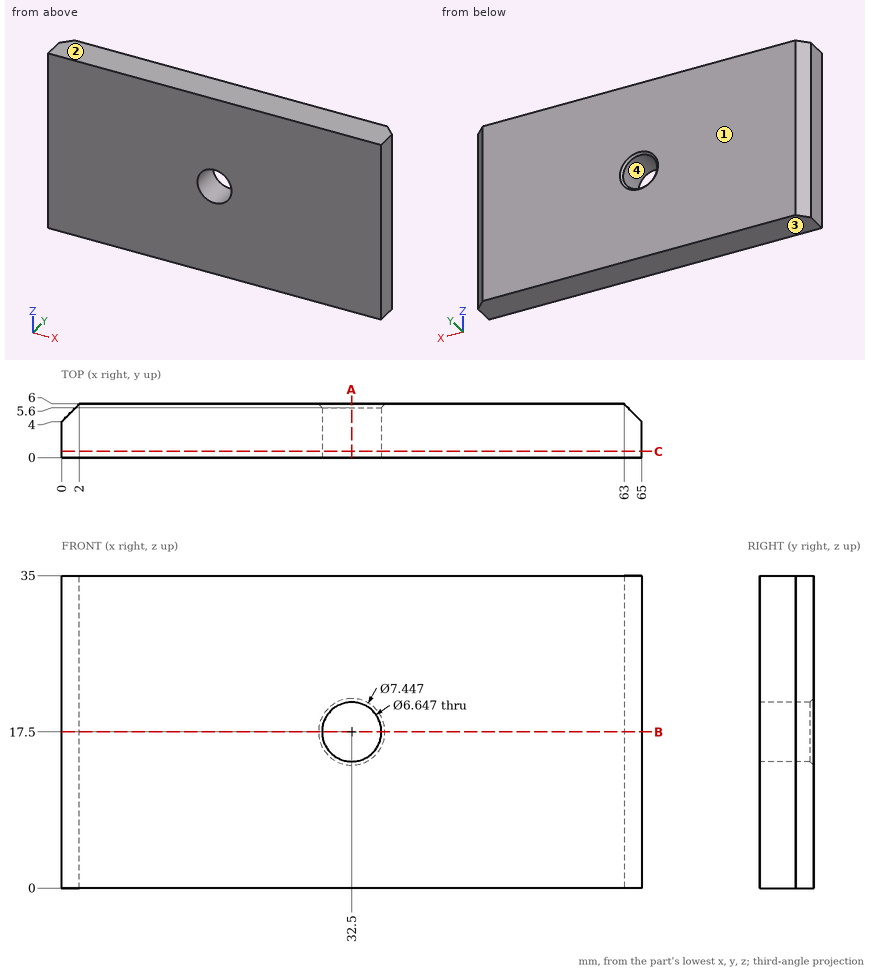
Study the drawing (mm; zero at the part's minimum x, y, z) and answer. Round coordinates to 2 decimals unless told otherwise and drop trailing zeros. Write each loop counter-clockwise with the first axis right and the second up, starting at its lowest first coordinate (ties: lowest second). Pieces come first, ordered by that corner, then holes.
1) A cutting plane is placed at A-A on x = 32.5. Determine the outline of the cut face in (y, z).
2) Determine the mould class of the marked faces 1, 2, 3 and 4 for opening direction Z: pulls with the +Z half, pulls with the -Z half, needs draft (parallel to the pull), parting line crosses it, or undercut.
3) A cutting plane is placed at C-C on y = 0.7. Determine the outline of the cut face in (x, z).
4) A cutting plane is placed at B-B on z = 17.5. Determine the outline of the cut face in (x, y).
5) Consider probe 1 along X at (y, z) = (2.3, 17.5); probe 2 along Z at (x, y) = (32.5, 4.4); probe 3 along X at (y, z) = (2.2, 15). Determine where each line is inside the solid, lowest interval first.
Entries:
1. outline: (0, 0) - (6, 0) - (6, 13.78) - (5.6, 14.18) - (0, 14.18) - close; (0, 20.82) - (5.6, 20.82) - (6, 21.22) - (6, 35) - (0, 35) - close
2. face 1: needs draft
2. face 2: pulls with the +Z half
2. face 3: pulls with the -Z half
2. face 4: undercut
3. outline: (0, 0) - (65, 0) - (65, 35) - (0, 35) - close; hole circle Ø6.65 at (32.5, 17.5)
4. outline: (0, 0) - (29.18, 0) - (29.18, 5.6) - (28.78, 6) - (2, 6) - (0, 4) - close; (35.82, 0) - (65, 0) - (65, 4) - (63, 6) - (36.22, 6) - (35.82, 5.6) - close
5. probe 1: x = 0 to 29.18, 35.82 to 65
5. probe 2: z = 0 to 14.18, 20.82 to 35
5. probe 3: x = 0 to 30.31, 34.69 to 65
